from build123d import *

# Parameters (mm, degrees)
SKETCH1_W           = 99
SKETCH1_H           = 199
BOSS_EXTRUDE1_DEPTH = 50
SKETCH2_W           = 96
SKETCH2_H           = 4
CUT_EXTRUDE1_DEPTH  = 48.5
BOSS_EXTRUDE2_REACH = 213.072
SKETCH7_W           = 58
SKETCH7_H           = 18.5
BOSS_EXTRUDE3_DEPTH = 11
SKETCH9_R           = 1.25
CUT_EXTRUDE6_DEPTH  = 131.432932958
SKETCH10_R          = 1.25
CUT_EXTRUDE7_DEPTH  = 5
CUT_EXTRUDE8_START  = -10
SKETCH11_R          = 1.25
CUT_EXTRUDE8_DEPTH  = 10


with BuildPart() as part:
    # Sketch1 → Boss-Extrude1 (new body)
    with BuildSketch(Plane.XY):
        Rectangle(SKETCH1_W, SKETCH1_H)
    extrude(amount=BOSS_EXTRUDE1_DEPTH)

    # Sketch2 → Cut-Extrude1 (cut)
    with BuildSketch(Plane.XY.offset(50)):
        with Locations((0, -97.5)):
            Rectangle(SKETCH2_W, SKETCH2_H)
    extrude(amount=-CUT_EXTRUDE1_DEPTH, mode=Mode.SUBTRACT)

    # Sketch3 → Boss-Extrude2 (add, up to next)
    with BuildSketch(Plane.XZ.offset(99.5), mode=Mode.PRIVATE) as boss_extrude2_sk1:
        Polygon((39, 1.5), (-43.455469088, 1.5), (-48, 1.5), (-48, 10.5), (-19, 10.5), (-19, 25.5), (39, 25.5), align=None)
    boss_extrude2_tool1 = extrude(boss_extrude2_sk1.sketch, amount=-BOSS_EXTRUDE2_REACH, mode=Mode.PRIVATE) - part.part
    add(boss_extrude2_tool1.solids().sort_by_distance((3.131579, -99.5, 12.315789))[0])

    # Sketch7 → Boss-Extrude3 (add)
    with BuildSketch(Plane.XZ.offset(99.5)):
        with Locations((10, 16.25)):
            Rectangle(SKETCH7_W, SKETCH7_H)
    extrude(amount=BOSS_EXTRUDE3_DEPTH)

    # Sketch9 → Cut-Extrude6 (cut, through all)
    with BuildSketch(Plane.XY.offset(1.5)):
        with Locations((11.5, -79.5)):
            Circle(SKETCH9_R)
        with Locations((-39.5, -79.5)):
            Circle(SKETCH9_R)
        with Locations((-39.5, 88.5)):
            Circle(SKETCH9_R)
        with Locations((39.5, 88.5)):
            Circle(SKETCH9_R)
    extrude(amount=-CUT_EXTRUDE6_DEPTH, mode=Mode.SUBTRACT)

    # Sketch10 → Cut-Extrude7 (cut)
    with BuildSketch(Plane(origin=(49.5, 0, 0), x_dir=(0, 0, -1), z_dir=(1, 0, 0))):
        with Locations((-37.5, 42.5)):
            Circle(SKETCH10_R)
        with Locations((-12.5, 42.5)):
            Circle(SKETCH10_R)
        with Locations((-25, -74.5)):
            Circle(SKETCH10_R)
        with Locations((-12.5, -74.5)):
            Circle(SKETCH10_R)
    extrude(amount=-CUT_EXTRUDE7_DEPTH, mode=Mode.SUBTRACT)

    # Sketch11 → Cut-Extrude8 (cut)
    with BuildSketch(Plane.ZY.offset(49.5).offset(CUT_EXTRUDE8_START)):
        with Locations(Location((12.5, -74.5, 0), (0, 0, 180))):
            Circle(SKETCH11_R)
        with Locations(Location((12.5, 42.5, 0), (0, 0, 180))):
            Circle(SKETCH11_R)
    extrude(amount=CUT_EXTRUDE8_DEPTH, mode=Mode.SUBTRACT)


solid = part.part
Geometry: final body of the model. Coordinates: model frame, mm. A direction names the side the tool comes from. Give positions to 0.01 mm unless a question says otherwise; leave off trailing zeros. Write each loop counter-clockwise with the first axis right and the second up, starting at its lowest first coordinate (ties: lowest second). Pieces come first, ordered by that corner, then holes. Notation, with made-up numbers: M 18.25,-17.75 L 77.25,-17.75 A13 cw 77.25,7.25 Z; hole C -5,-27.75 d3. An arc over 180 degrees is marked long. Answer in a Markdown table with one row per item. Add a question column.
(1) Section D-D on x = -26. Return loops of the section in (y, z), and give its area (3 significant figures).
(2) Section B-B on z = 18. Return loops of the section in (x, y).
(3) Ray query, line 1 (X direction, y = -79.5, z = 0.75); line 2 (Y direction, x = -47, z = 12.5); line 3 (Y direction, x = 40.5, z = 24). Return the intervals inside material, ascending.
(4) Reachability of faces 5 (the flat face through (48, -98, 26)), 6 (the flat face through (10, -110.5, 16)), 7 (the flat face through (10, -105, 7)) from +Z, -Z, +X, -X, +Y, -Y: full face, straight path, thin tool, end or side. Return the list, or none.
(5) First-contact query: pin 1 (2 mm diameter, centred on y = -74.5, z = 12.5, fed in from -X); pin 2 (3 mm diameter, centred on x = -34.5, y = -98, fed in from +Z); pin 3 (0.8 mm diameter, centred on y = 43, z = 37.5, fed in from +X). Flat tips, straight axial feed; report the tip coordinate or a pass-through.
(6) Section A-A on x = -43. Return loops of the section in (y, z), and give its area (3 significant figures).
(7) Mould query, pull axis X, two halves, no side actions, for faces 1 (the flat face through (49.5, -1, 25)), 2 (the flat face through (-19, -103, 16)), 3 (the flat face through (-49.5, -1, 25)), 4 (the flat face through (-1, 1, 0)). Classes: +X half, -X half, draft (parallel to the pull), parting line (faces both ways), or undercut.
(8) Section C-C on x = 7. Return loops of the section in (y, z).
Result set:
| question | item | result |
|---|---|---|
| 1 | outline | M -99.5,0 L 99.5,0 L 99.5,50 L -95.5,50 L -95.5,10.5 L -99.5,10.5 Z |
| 1 | area | 9,790 mm^2 |
| 2 | outline | M -49.5,-99.5 L -48,-99.5 L -48,-95.5 L -19,-95.5 L -19,-110.5 L 39,-110.5 L 39,-95.5 L 48,-95.5 L 48,-99.5 L 49.5,-99.5 L 49.5,99.5 L -49.5,99.5 Z |
| 3 | line 1 | x = -49.5 to -40.75, -38.25 to 10.25, 12.75 to 49.5 |
| 3 | line 2 | y = -95.5 to -75.75, -73.25 to 41.25, 43.75 to 99.5 |
| 3 | line 3 | y = -95.5 to 99.5 |
| 4 | face 5 | +Z, -Y |
| 4 | face 6 | +Z, -Z, +X, -X, -Y |
| 4 | face 7 | -Z, +X, -X, -Y |
| 5 | pin 1 | stops at x = -39.5 |
| 5 | pin 2 | stops at z = 10.5 |
| 5 | pin 3 | stops at x = 44.5 |
| 6 | outline | M -99.5,0 L 99.5,0 L 99.5,50 L -95.5,50 L -95.5,10.5 L -99.5,10.5 Z; hole C -74.5,12.5 d2.5; hole C 42.5,12.5 d2.5 |
| 6 | area | 9,780 mm^2 |
| 7 | face 1 | +X half |
| 7 | face 2 | undercut |
| 7 | face 3 | -X half |
| 7 | face 4 | draft |
| 8 | outline | M -110.5,7 L -99.5,7 L -99.5,0 L 99.5,0 L 99.5,50 L -95.5,50 L -95.5,25.5 L -110.5,25.5 Z |
